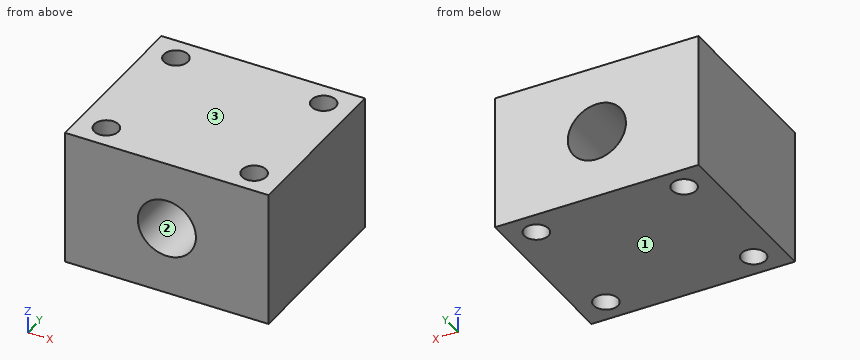
```python
from build123d import *

# Parameters (mm, degrees)
SKETCH_1_W               = 42
SKETCH_1_H               = 28
SKETCH_1_R               = 6
EXTRUDE_2_DEPTH          = 18
EXTRUDE_START            = -18
SKETCH_1_2_W             = 42
SKETCH_1_2_H             = 28
SKETCH_1_2_R             = 6
EXTRUDE_3_DEPTH          = 18
CUT_EXTRUDE_3_DEPTH      = 32
CUT_EXTRUDE_3_DEPTH_BACK = 32
SKETCH_3_R               = 2.5


with BuildPart() as part:
    # Sketch 1 → Extrude 2 (new body)
    with BuildSketch(Plane(origin=(0, 0, 0), x_dir=(1, 0, 0), z_dir=(0, 1, 0))):
        Rectangle(SKETCH_1_W, SKETCH_1_H)
        with Locations(Location((0, 0, 0), (0, 0, 270))):
            Circle(SKETCH_1_R, mode=Mode.SUBTRACT)
    extrude(amount=EXTRUDE_2_DEPTH)

    # Sketch 1_2 → Extrude 3 (add)
    with BuildSketch(Plane(origin=(0, 0, 0), x_dir=(1, 0, 0), z_dir=(0, 1, 0)).offset(EXTRUDE_START)):
        Rectangle(SKETCH_1_2_W, SKETCH_1_2_H)
        with Locations(Location((0, 0, 0), (0, 0, 270))):
            Circle(SKETCH_1_2_R, mode=Mode.SUBTRACT)
    extrude(amount=EXTRUDE_3_DEPTH)

    # Sketch 3 → Cut-Extrude 3 (cut, two sides: drawn at the far end of the back side and taken through both)
    with BuildSketch(Plane.XY.offset(-CUT_EXTRUDE_3_DEPTH_BACK)):
        with Locations((15.25, 13)):
            Circle(SKETCH_3_R)
        with Locations(Location((-15.25, 13, 0), (0, 0, 180))):
            Circle(SKETCH_3_R)
        with Locations(Location((15.25, -13, 0), (0, 0, 180))):
            Circle(SKETCH_3_R)
        with Locations((-15.25, -13)):
            Circle(SKETCH_3_R)
    extrude(amount=CUT_EXTRUDE_3_DEPTH + CUT_EXTRUDE_3_DEPTH_BACK, mode=Mode.SUBTRACT)


solid = part.part
```
Geometry check sheet. Reference: the model listing, model coordinates, mm. Face numbers are marked on the shaded views. Round coordinates to 2 decimals unless told otherwise and drop trailing zeros. Loops run counter-clockwise (first coordinate to the right, second up) from the corner with the lowest first, then second, coordinate; pieces in that order, holes last. Notation, with made-up numbers: (-11, -18) - (0, -18) arc R29 ccw to (0, 8) - close; hole circle Ø11 at (55.25, -1). An arc over 180 degrees is marked (long way). Write each question's results on one line, items separated by ' | '. Start each with the question number.
Q1. Cross-section at D-D on y = -8. Enter the section's corners in (x, z).
Q2. Release check for a two-part mould opening along Z. For the marked faces 1, 2 and 3 record: +Z half, -Z half, draft (parallel to the pull), parting line (faces both ways), or undercut.
Q3. Cross-section at C-C on y = -13. Enter the section's corners in (x, z), and give its area (3 significant figures).
Q4. Cross-section at A-A on z = 0. Enter the section's corners in (x, y).
Q5. Cross-section at B-B on x = 0. Enter the section's corners in (y, z).
Q6. Thickness scan on line 1 (Y direction, x = -15.25, z = -4.25); line 2 (Y direction, x = -13.5, z = -4.75); line 3 (X direction, y = 11, z = -4). Record the ranges inside material, lowest first. Write a range as [from, to].
Q7. Gauge pin test, flat ends, axial feed: P1, Ø6, axis at x = 15.25, y = 13, coming from the -Z side; P2, Ø3, axis at x = -15.25, y = -13, coming from the +Z side. Record the tip position at first contact, or that the pin passes through.
Answers below:
1) outline: (-21, -14) - (21, -14) - (21, 14) - (-21, 14) - close; hole circle Ø12 at (0, 0)
2) face 1: -Z half | face 2: undercut | face 3: +Z half
3) outline: (-21, -14) - (-17.75, -14) - (-17.75, 14) - (-21, 14) - close; (-12.75, -14) - (12.75, -14) - (12.75, 14) - (-12.75, 14) - close; (17.75, -14) - (21, -14) - (21, 14) - (17.75, 14) - close; hole circle Ø12 at (0, 0) | area: 783 mm²
4) outline: (-21, -18) - (-6, -18) - (-6, 18) - (-21, 18) - close; (6, -18) - (21, -18) - (21, 18) - (6, 18) - close; hole circle Ø5 at (-15.25, -13); hole circle Ø5 at (-15.25, 13); hole circle Ø5 at (15.25, -13); hole circle Ø5 at (15.25, 13)
5) outline: (-18, -14) - (18, -14) - (18, -6) - (-18, -6) - close; (-18, 6) - (18, 6) - (18, 14) - (-18, 14) - close
6) line 1: y = [-18, -15.5], [-10.5, 10.5], [15.5, 18] | line 2: y = [-18, -14.79], [-11.21, 11.21], [14.79, 18] | line 3: x = [-21, -16.75], [-13.75, -4.47], [4.47, 13.75], [16.75, 21]
7) P1: stops at z = -14 | P2: passes through
